```python
from build123d import *

# Parameters (mm, degrees)
SKETCH1_R               = 60
BOSS_EXTRUDE1_DEPTH     = 150
CUT_EXTRUDE1_DEPTH      = 173.336879396
CUT_EXTRUDE1_DEPTH_BACK = 173.336879396
SKETCH2_W               = 70
SKETCH2_H               = 100
FILLET1_R               = 10
CUT_EXTRUDE2_DEPTH      = 173.336879553
CUT_EXTRUDE2_DEPTH_BACK = 173.336879553
SKETCH3_OUTSIDE_W       = 167.3
SKETCH3_OUTSIDE_H       = 197.3
CUT_EXTRUDE3_DEPTH      = 199.305320239
CUT_EXTRUDE3_DEPTH_BACK = 199.305320239
SKETCH4_R               = 15
CIRPATTERN1_COUNT       = 4
CHAMFER1_SIZE           = 8
HOLE1_D                 = 14.5
HOLE1_CBORE_D           = 20
HOLE1_CBORE_DEPTH       = 25
CHAMFER3_SIZE           = 1
CHAMFER4_SIZE           = 1


with BuildPart() as part:
    # Sketch1 → Boss-Extrude1 (new body)
    with BuildSketch(Plane(origin=(0, 0, 0), x_dir=(1, 0, 0), z_dir=(0, 1, 0))):
        with Locations(Location((0, 0, 0), (0, 0, 270))):
            Circle(SKETCH1_R)
    extrude(amount=BOSS_EXTRUDE1_DEPTH)

    # Sketch2 → Cut-Extrude1 (cut, two sides: drawn at the far end of the back side and taken through both)
    with BuildSketch(Plane.XY.offset(-CUT_EXTRUDE1_DEPTH_BACK)):
        with Locations((0, 100)):
            Rectangle(SKETCH2_W, SKETCH2_H)
        Polygon((-55, 150), (-55, 80), (-60, 71.339745962), (-60, 150), align=None)
        Polygon((55, 80), (60, 71.339745962), (60, 150), (55, 150), align=None)
    extrude(amount=CUT_EXTRUDE1_DEPTH + CUT_EXTRUDE1_DEPTH_BACK, mode=Mode.SUBTRACT)

    # Fillet1
    fillet1_edges = [part.edges().sort_by_distance(p)[0] for p in [
        (-35, 50, 0),
        (35, 50, 0),
        (-55, 80, 0),
        (55, 80, 0),
    ]]
    fillet(fillet1_edges, radius=FILLET1_R)

    # Sketch3 outside → Cut-Extrude2 (cut, two sides: drawn at the far end of the back side and taken through both)
    with BuildSketch(Plane(origin=(0, 0, 0), x_dir=(0, 0, -1), z_dir=(1, 0, 0)).offset(-CUT_EXTRUDE2_DEPTH_BACK)):
        with Locations((0, 75)):
            Rectangle(SKETCH3_OUTSIDE_W, SKETCH3_OUTSIDE_H)
        with BuildLine():
            Line((-12.5, 150), (-30, 132.5))
            Line((-30, 132.5), (-30, 40.886751346))
            ThreePointArc((-30, 40.886751346), (-30.669872981, 38.386751346), (-32.5, 36.556624327))
            Line((-32.5, 36.556624327), (-60, 20.679491924))
            Line((-60, 20.679491924), (-60, 0))
            Line((-60, 0), (60, 0))
            Line((60, 0), (60, 20.679491924))
            Line((60, 20.679491924), (32.5, 36.556624327))
            ThreePointArc((32.5, 36.556624327), (30.669872981, 38.386751346), (30, 40.886751346))
            Line((30, 40.886751346), (30, 132.5))
            Line((30, 132.5), (12.5, 150))
            Line((12.5, 150), (-12.5, 150))
        make_face(mode=Mode.SUBTRACT)
    extrude(amount=CUT_EXTRUDE2_DEPTH + CUT_EXTRUDE2_DEPTH_BACK, mode=Mode.SUBTRACT)

    # Sketch4 → Cut-Extrude3 (cut, two sides: drawn at the far end of the back side and taken through both)
    with BuildSketch(Plane(origin=(55, 0, 0), x_dir=(0, 0, -1), z_dir=(1, 0, 0)).offset(-CUT_EXTRUDE3_DEPTH_BACK)):
        with Locations(Location((0, 120, 0), (0, 0, 90))):
            Circle(SKETCH4_R)
    extrude(amount=CUT_EXTRUDE3_DEPTH + CUT_EXTRUDE3_DEPTH_BACK, mode=Mode.SUBTRACT)

    # Sketch6 → M5 Tapped Hole1 (revolve, cut)
    with BuildSketch(Plane(origin=(55, 135.909902577, -15.909902577), x_dir=(0, 0, -1), z_dir=(0, 1, 0))):
        Polygon((0, 0), (0, 17.2618073), (2.1, 16), (2.1, 0), align=None)
    m5_tapped_hole1 = revolve(axis=Axis((61.35, 135.909902577, -15.909902577), (-1, 0, 0)), mode=Mode.SUBTRACT)

    # CirPattern1: M5 Tapped Hole1 ×4 about axis
    cirpattern1_axis = Axis((0, 120, 0), (1, 0, 0))
    for i in range(1, CIRPATTERN1_COUNT):
        add(m5_tapped_hole1.rotate(cirpattern1_axis, i * 360 / CIRPATTERN1_COUNT), mode=Mode.SUBTRACT)

    # Mirror1: M5 Tapped Hole1 across plane
    add(m5_tapped_hole1.mirror(Plane(origin=(0, 0, 0), x_dir=(0, 0, 1), z_dir=(1, 0, 0))), mode=Mode.SUBTRACT)

    # Mirror1 copy 1 sketch → Mirror1 copy 1 (revolve, cut)
    with BuildSketch(Plane(origin=(-55, 135.909902577, 15.909902577), x_dir=(0, 1, 0), z_dir=(0, 0, 1))):
        Polygon((0, 0), (0, -17.2618073), (2.1, -16), (2.1, 0), align=None)
    revolve(axis=Axis((-61.35, 135.909902577, 15.909902577), (-1, 0, 0)), mode=Mode.SUBTRACT)

    # Mirror1 copy 2 sketch → Mirror1 copy 2 (revolve, cut)
    with BuildSketch(Plane(origin=(-55, 104.090097423, 15.909902577), x_dir=(0, 0, 1), z_dir=(0, -1, 0))):
        Polygon((0, 0), (0, -17.2618073), (2.1, -16), (2.1, 0), align=None)
    revolve(axis=Axis((-61.35, 104.090097423, 15.909902577), (-1, 0, 0)), mode=Mode.SUBTRACT)

    # Mirror1 copy 3 sketch → Mirror1 copy 3 (revolve, cut)
    with BuildSketch(Plane(origin=(-55, 104.090097423, -15.909902577), x_dir=(0, -1, 0), z_dir=(0, 0, -1))):
        Polygon((0, 0), (0, -17.2618073), (2.1, -16), (2.1, 0), align=None)
    revolve(axis=Axis((-61.35, 104.090097423, -15.909902577), (-1, 0, 0)), mode=Mode.SUBTRACT)

    # Chamfer1
    chamfer1_edges = [part.edges().sort_by_distance(p)[0] for p in [
        (32.071067812, 52.928932188, 30),
        (32.071067812, 52.928932188, -30),
        (-35, 150, 0),
        (35, 150, 0),
        (35, 141.25, -21.25),
        (-35, 141.25, -21.25),
        (35, 141.25, 21.25),
        (-35, 141.25, 21.25),
        (-35, 96.25, -30),
        (-32.071067812, 52.928932188, -30),
        (0, 50, -30),
        (35, 96.25, -30),
        (-32.071067812, 52.928932188, 30),
        (-35, 96.25, 30),
        (35, 96.25, 30),
        (0, 50, 30),
    ]]
    chamfer(chamfer1_edges, length=CHAMFER1_SIZE)

    # Hole1 (through all)
    with Locations(Plane(origin=(-27, 50, -43), x_dir=(1, 0, 0), z_dir=(0, 1, 0))):
        with Locations((0, 0), (54, 0), (0, -86), (54, -86)):
            CounterBoreHole(HOLE1_D / 2, HOLE1_CBORE_D / 2, HOLE1_CBORE_DEPTH)

    # Chamfer3
    chamfer3_edges = [part.edges().sort_by_distance(p)[0] for p in [
        (0, 0, -60),
    ]]
    chamfer(chamfer3_edges, length=CHAMFER3_SIZE)

    # Chamfer4
    chamfer4_edges = [part.edges().sort_by_distance(p)[0] for p in [
        (55, 105, 0),
        (-55, 105, 0),
    ]]
    chamfer(chamfer4_edges, length=CHAMFER4_SIZE)

    # Chamfer5
    # the kernel refuses this chamfer: 2 mm, written as the material it takes off along each edge
    with BuildSketch(Plane(origin=(35.377389831, 32.524460395, -48.460708711), x_dir=(0.7977683815580907, 0, 0.6029640199764695), z_dir=(0, -1, 0))) as chamfer5_piece_1:
        with BuildLine():
            Line((1.994201413, 0), (1.846539445, 0.888707135))
            ThreePointArc((1.846539445, 0.888707135), (0.956280866, 0.401837503), (0, 0))
            ThreePointArc((0, 0), (1.003653566, -0.008285296), (1.994201413, 0))
        make_face()
    extrude(amount=7.524460395, mode=Mode.SUBTRACT)
    with BuildSketch(Plane(origin=(-35.377389831, 32.524460395, -48.460708711), x_dir=(-0.7977683815580952, 0, 0.602964019976464), z_dir=(0, -1, 0))) as chamfer5_piece_2:
        with BuildLine():
            Line((1.994201413, 0), (1.846539445, -0.888707135))
            ThreePointArc((1.846539445, -0.888707135), (0.956280866, -0.401837503), (0, 0))
            ThreePointArc((0, 0), (1.003653566, 0.008285296), (1.994201413, 0))
        make_face()
    extrude(amount=7.524460395, mode=Mode.SUBTRACT)

    # Chamfer6
    # the kernel refuses this chamfer: 2 mm, written as the material it takes off along each edge
    with BuildSketch(Plane(origin=(-35.377389831, 32.524460395, 48.460708711), x_dir=(-0.45735909504580285, 0, -0.8892821026979484), z_dir=(0, -1, 0))) as chamfer6_piece_1:
        with BuildLine():
            Line((2.049270186, 0), (1.79691853, -0.864825457))
            ThreePointArc((1.79691853, -0.864825457), (0.900770777, -0.442720154), (0, 0))
            ThreePointArc((0, 0), (1.035942557, -0.052625969), (2.049270186, 0))
        make_face()
    extrude(amount=7.524460395, mode=Mode.SUBTRACT)
    with BuildSketch(Plane(origin=(35.377389831, 32.524460395, 48.460708711), x_dir=(0.45735909504580835, 0, -0.8892821026979455), z_dir=(0, -1, 0))) as chamfer6_piece_2:
        with BuildLine():
            Line((2.049270186, 0), (1.79691853, 0.864825457))
            ThreePointArc((1.79691853, 0.864825457), (0.900770777, 0.442720154), (0, 0))
            ThreePointArc((0, 0), (1.035942557, 0.052625969), (2.049270186, 0))
        make_face()
    extrude(amount=7.524460395, mode=Mode.SUBTRACT)

    # Sketch12 → Cut-Revolve1 (revolve, cut)
    with BuildSketch(Plane.XY):
        Polygon((37, 147.5), (37, 120), (32, 120), (32, 152.5), align=None)
    cut_revolve1 = revolve(axis=Axis((37, 120, 0), (-1, 0, 0)), mode=Mode.SUBTRACT)

    # Mirror2: Cut-Revolve1 across plane
    add(cut_revolve1.mirror(Plane(origin=(0, 0, 0), x_dir=(0, 0, 1), z_dir=(1, 0, 0))), mode=Mode.SUBTRACT)


solid = part.part
```
Geometry check sheet. Reference: the model listing, model coordinates, mm. A direction names the side the tool comes from. Coordinates: 2 decimals unless noted, no trailing zeros. Order: outer loops, then holes, each group sorted by start corner. A loop starts at its lowest first (then second) coordinate and runs counter-clockwise, first axis right, second up.
Q1. Depth check by flat-ended pin: pin 1 Ø8 at (x, y) = (-22, 28) entering from +Z; pin 2 Ø12 at (x, z) = (43, 19) entering from -Y; pin 3 Ø10 at (x, z) = (-29.5, 40) entering from +Y; pin 4 Ø5 at (y, z) = (135.91, -15.91) entering from +X. Enter the tip coordinate at first touch or a pass-through.
Reply:
pin 1: stops at z = 54.25
pin 2: stops at y = 0
pin 3: stops at y = 25
pin 4: stops at x = 55
Q2. Tool access check on faces 4 (the face through (-28.203, 29.543, -33.073)), 5 (the face through (-34.332, 50.871, -25.055)), 6 (the face through (-46, 76, -30)). Record the directions out of +Z, -Z, +X, -X, +Y, -Y that give a thin tool (end or side, any length) a straight path to the whole face; none if there is none.
Reply:
face 4: +Y
face 5: -Z, +Y
face 6: -Z, +X, -X, +Y
Q3. Sectioned sample at C-C on x = 0. Record the cut outline in (y, z).
Reply:
outline: (0, -59) - (1, -60) - (20.68, -60) - (36.56, -32.5) arc R5 cw to (40.89, -30) - (42, -30) - (50, -22) - (50, 22) - (42, 30) - (40.89, 30) arc R5 cw to (36.56, 32.5) - (20.68, 60) - (1, 60) - (0, 59) - close
Q4. Sectioned sample at D-D on z = 0. Give the number of separate pieces and of enclosed holes in the cut face, and give its area (3 significant figures).
Reply:
separate pieces: 3
enclosed holes: 0
area: 8,950 mm2
Q5. Thickness scan on probe 1 along X at (y, z) = (100, -0.5); probe 2 along Y at (x, z) = (47.5, 0); probe 3 along Z at (x, y) = (27, 7). Record the ranges inside material, lowest first.
Reply:
probe 1: x = -55 to -37, 37 to 55
probe 2: y = 0 to 105, 135 to 150
probe 3: z = -53.58 to -50.25, -35.75 to 35.75, 50.25 to 53.58
Q6. Sectioned sample at B-B on y = 63. Record the cut outline in (x, z).
Reply:
outline: (-51.96, -30) - (-43, -30) - (-35, -22) - (-35, 22) - (-43, 30) - (-51.96, 30) arc R60 ccw to start; (35, -22) - (43, -30) - (51.96, -30) arc R60 ccw to (51.96, 30) - (43, 30) - (35, 22) - close
Q7. Draft check along X on faces 1 (the face through (-49.1, 141.1, -21.4)), 2 (the face through (37.957, 103.767, 16.078)), 3 (the face through (-34, 25, 40)). Enter one of: released by +X, released by -X, zero draft, split by the parting line, or undercut.
Reply:
face 1: zero draft
face 2: released by +X
face 3: undercut
Q8. Sectioned sample at A-A on y = 120. Record the cut outline in (x, z).
Reply:
outline: (-55, -23.98) arc R60 ccw to (-51.96, -30) - (-43, -30) - (-37, -24) - (-37, -15) - (-54, -15) - (-55, -16) - close; (-55, 16) - (-54, 15) - (-37, 15) - (-37, 24) - (-43, 30) - (-51.96, 30) arc R60 ccw to (-55, 23.98) - close; (37, -24) - (43, -30) - (51.96, -30) arc R60 ccw to (55, -23.98) - (55, -16) - (54, -15) - (37, -15) - close; (37, 15) - (54, 15) - (55, 16) - (55, 23.98) arc R60 ccw to (51.96, 30) - (43, 30) - (37, 24) - close
